```python
from build123d import *

# Parameters (mm, degrees)
F0_R     = 38.1
F1_DEPTH = 4.318
F3_DEPTH = 2.54
F4_R     = 36.159311
F5_DEPTH = 2.54


with BuildPart() as f1:
    # F0 (on Top) → F1 (new body)
    with BuildSketch(Plane.XY):
        Circle(F0_R)
    extrude(amount=F1_DEPTH)

    # F2 (on face) → F3 (join)
    with BuildSketch(Plane.XY.offset(4.318)):
        Polygon((-34.062076, 12.440001), (-7.371115, -14.31433), (-7.371115, -18.005043), (-9.246102, -18.000251), (-9.246102, -21.084584), (-8.250766, -20.103207), (-6.302369, -20.103207), (-6.302369, -21.906156), (-7.371115, -22.959914), (-4.425159, -22.959914), (-3.651459, -24.593657), (-3.340078, -25.019994), (0.323527, -27.597751), (3.852937, -25.019994), (4.285339, -24.593657), (5.079073, -22.959914), (8.107178, -22.959914), (7.050497, -21.906156), (7.050497, -20.103207), (8.963848, -20.103207), (9.898308, -21.094017), (9.898308, -18.005043), (8.015761, -18.005043), (8.015761, -14.323118), (34.762263, 12.40246), (14.500252, 12.40246), (9.73234, 7.673752), (9.73234, 2.785812), (8.937273, 1.987536), (4.18791, 1.987536), (4.18791, 5.622365), (6.957923, 8.360175), (6.957923, 8.555209), (4.987081, 8.555209), (3.098329, 6.672881), (2.346354, 6.672881), (2.346354, 7.621024), (5.079073, 10.368997), (6.00274, 10.368997), (6.00274, 10.558032), (4.160542, 12.40246), (2.923493, 12.40246), (0.086455, 9.55383), (-2.58904, 9.55383), (-3.608238, 8.555209), (-3.608238, 1.95247), (-8.261997, 1.95247), (-9.084493, 2.805168), (-9.084493, 7.649168), (-13.932226, 12.440001), align=None)
        Polygon((-6.296679, -10.668362), (-6.296679, -0.112185), (-4.45952, -1.943368), (-1.514731, -1.943368), (0.321967, -0.112185), (2.1779, -1.943368), (5.056894, -1.943368), (6.863146, -0.112185), (6.863146, -10.668362), (5.965335, -12.48001), (3.199338, -15.198641), (1.351123, -16.080152), (0.252056, -17.160398), (-0.809691, -16.080152), (-2.588448, -15.198641), (-5.260525, -12.48001), align=None, mode=Mode.SUBTRACT)
        Polygon((-1.665403, -11.440925), (4.168083, -5.593271), (4.168083, -3.724239), (2.277503, -3.724239), (-3.569818, -9.596433), (-3.569818, -11.440925), align=None)
    extrude(amount=F3_DEPTH)

    # F4 (on Top) → F5 (join)
    with BuildSketch(Plane.XY):
        Circle(F4_R)
        with BuildLine():
            ThreePointArc((5.794921, -30.256666), (-23.744145, 19.628106), (30.806606, 0))
            ThreePointArc((30.806606, 0), (28.080712, -12.669672), (20.385426, -23.097216))
            ThreePointArc((20.385426, -23.097216), (13.570817, -27.656462), (5.794921, -30.256666))
        make_face(mode=Mode.SUBTRACT)
        with BuildLine():
            Line((0, -22.444444), (5.794921, -30.256666))
            ThreePointArc((5.794921, -30.256666), (13.570817, -27.656462), (20.385426, -23.097216))
            Line((20.385426, -23.097216), (13.933389, -16.605597))
            Line((13.933389, -16.605597), (8.745673, -11.386055))
            Line((8.745673, -11.386055), (7.496308, -12.30919))
            Line((7.496308, -12.30919), (3.57206, -6.998139))
            Line((3.57206, -6.998139), (4.371937, -1.893155))
            Line((4.371937, -1.893155), (1.590109, 1.871753))
            Line((1.590109, 1.871753), (11.763458, 11.98307))
            Line((11.763458, 11.98307), (18.729663, 4.974128))
            Line((18.729663, 4.974128), (21.665659, 7.892222))
            Line((21.665659, 7.892222), (15.77972, 16.543103))
            Line((15.77972, 16.543103), (17.309812, 18.063865))
            Line((17.309812, 18.063865), (13.368929, 22.028926))
            Line((13.368929, 22.028926), (11.763458, 20.433245))
            Line((11.763458, 20.433245), (4.110456, 28.133198))
            Line((4.110456, 28.133198), (-0.682113, 23.369851))
            Line((-0.682113, 23.369851), (7.16014, 15.479486))
            Line((7.16014, 15.479486), (-3.149464, 5.232744))
            Line((-3.149464, 5.232744), (-6.889652, 7.478646))
            Line((-6.889652, 7.478646), (-9.403128, 6.031075))
            Line((-9.403128, 6.031075), (-9.92541, 4.087029))
            Line((-9.92541, 4.087029), (-12.478785, 2.839357))
            Line((-12.478785, 2.839357), (-13.059097, 0.808264))
            Line((-13.059097, 0.808264), (-15.003144, -0.468424))
            Line((-15.003144, -0.468424), (-15.003144, -1.251846))
            Line((-15.003144, -1.251846), (-16.387494, -3.31088))
            Line((-16.387494, -3.31088), (-14.87847, -6.998139))
            Line((-14.87847, -6.998139), (-18.722013, -10.818246))
            Line((-18.722013, -10.818246), (-14.710922, -14.853945))
            Line((-14.710922, -14.853945), (-11.050018, -11.215364))
            Line((-11.050018, -11.215364), (-8.104812, -14.178638))
            Line((-8.104812, -14.178638), (-4.658059, -15.363094))
            Line((-4.658059, -15.363094), (0.897256, -21.77888))
            Line((0.897256, -21.77888), (0, -22.444444))
        make_face()
    extrude(amount=-F5_DEPTH)


solid = f1.part
```
Geometry check sheet. Reference: the model listing, model coordinates, mm. A direction names the side the tool comes from. Round coordinates to 2 decimals unless told otherwise and drop trailing zeros. Order: outer loops, then holes, each group sorted by start corner. A loop starts at its lowest first (then second) coordinate and runs counter-clockwise, first axis right, second up. Notation, with made-up numbers: (22.25, 36) -> (27.25, 36) arc R17 cw to (27.25, 67) -> close; hole circle Ø7 at (41.25, 28). An arc over 180 degrees is marked (long way). Return JSON: item names as keys, results as strings. Group by question number.
Q1. Gauge pin test, flat ends, axial feed: pin 1 (5 mm diameter, centred on y = 30, z = -0.5, fed in from +X); pin 2 (0.7 mm diameter, centred on x = 5.5, z = 5.5, fed in from -Y); pin 3 (1 mm diameter, centred on x = -6.5, y = 16.5, fed in from +Z); pin 4 (23 mm diameter, centred on x = -8.5, y = 9, fed in from -Z). Record the tip position at first contact, or that the pin passes through.
Q2. Tool access check on faces 5 (the flat face through (3.184, 19.48, -1.252)), 6 (the flat face through (6.4, -11.6, 5.6)), 7 (the flat face through (-7.371, -16, 6)). Record the directions out of +Z, -Z, +X, -X, +Y, -Y that give a thin tool (end or side, any length) a straight path to the whole face; none if there is none.
Q3. Section check C-C, the plane z = 3. Record the boundary of the cut face in (x, y), plus the area to 3 significant figures.
Q4. Release check for a two-part mould opening along Y. For faces 1 (the flat face through (-4.99, 6.34, -1.25)), 2 (the flat face through (2, -9, 4.318)), 3 (the flat face through (4.677, -23.788, 5.57)), 4 (the flat face through (3, 1, 6.858)) record: released by +Y, released by -Y, zero draft, split by the parting line, or undercut.
Q5. Section check A-A, the plane x = 29.5. Record the boundary of the cut face in (y, z), plus the area to 3 significant figures.
Q6. Material ranges on probe 1 along Y at (x, z) = (4.5, -1.25); probe 2 along Z at (x, y) = (-29.5, -6); probe 3 along Z at (x, y) = (-9, 6), recorded low to high. Write a range as from..to.
Q7. Section check B-B, the plane y = 27. Record the boundary of the cut face in (x, z).
Numbers:
{
 "1": {"pin 1": "x = 26.32", "pin 2": "y = -22.96", "pin 3": "z = 4.32", "pin 4": "z = -2.54"},
 "2": {"face 5": "-Z", "face 6": "+Z", "face 7": "+Z, -X"},
 "3": {"outline": "circle Ø76.2 at (0, 0)", "area": "4,560 mm^2"},
 "4": {"face 1": "undercut", "face 2": "undercut", "face 3": "released by -Y", "face 4": "zero draft"},
 "5": {"outline": "(-24.11, 0) -> (-20.91, 0) -> (-20.91, -2.54) -> (-8.88, -2.54) -> (-8.88, 0) -> (8.88, 0) -> (8.88, -2.54) -> (20.91, -2.54) -> (20.91, 0) -> (24.11, 0) -> (24.11, 4.32) -> (12.4, 4.32) -> (12.4, 6.86) -> (7.14, 6.86) -> (7.14, 4.32) -> (-24.11, 4.32) -> close", "area": "283 mm^2"},
 "6": {"probe 1": "-35.88..-30.48, -28.51..-8.25, 4.76..12.84, 18.16..27.74, 30.48..35.88", "probe 2": "0..4.32", "probe 3": "-2.54..4.32"},
 "7": {"outline": "(-26.88, 0) -> (-24.05, 0) -> (-24.05, -2.54) -> (-14.83, -2.54) -> (-14.83, 0) -> (2.97, 0) -> (2.97, -2.54) -> (5.24, -2.54) -> (5.24, 0) -> (14.83, 0) -> (14.83, -2.54) -> (24.05, -2.54) -> (24.05, 0) -> (26.88, 0) -> (26.88, 4.32) -> (-26.88, 4.32) -> close"}
}
